CAD build for the part. Positions are in the model's coordinates, mm. A direction names the side the tool comes from. Give positions to 0.01 mm unless a question says otherwise; leave off trailing zeros. Write each loop counter-clockwise with the first axis right and the second up, starting at its lowest first coordinate (ties: lowest second). Pieces come first, ordered by that corner, then holes. Notation, with made-up numbers: (84.25, 79.5) -> (137.25, 79.5) arc R36 cw to (137.25, 115.5) -> close; hole circle Ø9 at (11, -33). An arc over 180 degrees is marked (long way). Answer as a JSON object with one key per item and string values.
```python
from build123d import *

# Parameters (mm, degrees)
F1_DEPTH = 20
F3_DEPTH = 3
F4_R     = 1


with BuildPart() as f1:
    # F0 (on Top) → F1 (new body)
    with BuildSketch(Plane.XY):
        with BuildLine():
            ThreePointArc((-22.105041, 11.299526), (-27.279634, -7.687217), (-7.672847, -6))
            Line((-7.672847, -6), (7.672847, -6))
            ThreePointArc((7.672847, -6), (27.279634, -7.687217), (22.105041, 11.299526))
            ThreePointArc((22.105041, 11.299526), (18.842402, 11.974802), (15.519847, 11.726953))
            ThreePointArc((15.519847, 11.726953), (10.990907, 9.693042), (7.672847, 6))
            Line((7.672847, 6), (-1.3, 6))
            Line((-1.3, 6), (-7.672847, 6))
            ThreePointArc((-7.672847, 6), (-10.990907, 9.693042), (-15.519847, 11.726953))
            ThreePointArc((-15.519847, 11.726953), (-18.842402, 11.974802), (-22.105041, 11.299526))
        make_face()
        with BuildLine():
            Line((-8.9, 4), (0, 4))
            Line((0, 4), (8.9, 4))
            ThreePointArc((8.9, 4), (28.065151, 0), (8.9, -4))
            Line((8.9, -4), (-8.9, -4))
            ThreePointArc((-8.9, -4), (-28.065151, 0), (-8.9, 4))
        make_face(mode=Mode.SUBTRACT)
        with BuildLine():
            ThreePointArc((22.105041, 11.299526), (0, 15.132305), (-22.105041, 11.299526))
            ThreePointArc((-22.105041, 11.299526), (-18.842402, 11.974802), (-15.519847, 11.726953))
            ThreePointArc((-15.519847, 11.726953), (0, 13.632305), (15.519847, 11.726953))
            ThreePointArc((15.519847, 11.726953), (18.842402, 11.974802), (22.105041, 11.299526))
        make_face()
    extrude(amount=F1_DEPTH)

    # F2 (on face) → F3 (join)
    with BuildSketch(Plane.XZ.offset(6)):
        Polygon((1.5, 20), (0, 20), (-1.5, 20), (-1.5, 0), (0, 0), (1.5, 0), align=None)
    extrude(amount=F3_DEPTH)

    # F4
    f4_edges = [f1.edges().sort_by_distance(p)[0] for p in [
        (1.5, -9, 10),
        (-1.5, -9, 10),
    ]]
    fillet(f4_edges, radius=F4_R)


solid = f1.part
```
1) Slice it at C-C (z = 9.25). List the corners of the cut face in (x, y), then the cut area to 3 significant figures.
Model answer:
{"outline": "(-22.11, 11.3) arc R12 ccw (long way) to (-7.67, -6) -> (-1.5, -6) -> (-1.5, -8) arc R1 ccw to (-0.5, -9) -> (0.5, -9) arc R1 ccw to (1.5, -8) -> (1.5, -6) -> (7.67, -6) arc R12 ccw (long way) to (22.11, 11.3) arc R65.66 ccw to start; hole (-15.52, 11.73) arc R12 cw to (-7.67, 6) -> (7.67, 6) arc R12 cw to (15.52, 11.73) arc R64.16 ccw to start; hole (-8.9, -4) -> (8.9, -4) arc R10 ccw (long way) to (8.9, 4) -> (-8.9, 4) arc R10 ccw (long way) to start", "area": "364 mm2"}
2) Slice it at D-D (y = -5). List the corners of the cut face in (x, z), then the cut area to 3 significant figures.
Model answer:
{"outline": "(-28.97, 0) -> (-26.73, 0) -> (-26.73, 20) -> (-28.97, 20) -> close; (-9.4, 0) -> (9.4, 0) -> (9.4, 20) -> (-9.4, 20) -> close; (26.73, 0) -> (28.97, 0) -> (28.97, 20) -> (26.73, 20) -> close", "area": "466 mm2"}
3) Slice it at B-B (x = 6). List the corners of the cut face in (y, z).
Model answer:
{"outline": "(-6, 0) -> (-4, 0) -> (-4, 20) -> (-6, 20) -> close; (4, 0) -> (6, 0) -> (6, 20) -> (4, 20) -> close; (13.35, 0) -> (14.86, 0) -> (14.86, 20) -> (13.35, 20) -> close"}
4) Mould opens along Y. For faces 4 (the cylindrical face through (-27.48, -7.44, 9.86)), 5 (the flat face through (5, -6, 10)), 6 (the flat face through (0, -4, 10)), 7 (the flat face through (0, 5, 0)) say: released by +Y, released by -Y, zero draft, split by the parting line, or undercut.
Model answer:
{"face 4": "split by the parting line", "face 5": "released by -Y", "face 6": "undercut", "face 7": "zero draft"}
5) Pin check, flat tips, straight feed: pin 1 (16 mm diameter, centred on x = -18.07, y = 0, fed in from +Z); pin 2 (6 mm diameter, centred on y = 6, z = 16.5, fed in from -X); pin 3 (3 mm diameter, centred on x = -10.5, z = 12.5, fed in from +Y); pin 4 (2 mm diameter, centred on y = -7.5, z = 8.5, fed in from -X). Stop position of each tip, or through.
Model answer:
{"pin 1": "passes through", "pin 2": "stops at x = -29.68", "pin 3": "stops at y = 14.51", "pin 4": "stops at x = -28.15"}
6) 3-axis set-ups, long thin cutter, end or side, ignore diameter. For faces 1 (the flat face through (0, 5, 20)), 2 (the flat face through (0, 4, 10)), 3 (the flat face through (-1.5, -7, 10)): which of +Z, -Z, +X, -X, +Y, -Y reach the whole face in a straight line?
Model answer:
{"face 1": "+Z, +X, -X, +Y, -Y", "face 2": "+Z, -Z", "face 3": "+Z, -Z, -Y"}
7) Slice it at A-A (y = 0). List the corners of the cut face in (x, z).
Model answer:
{"outline": "(-30.07, 0) -> (-28.07, 0) -> (-28.07, 20) -> (-30.07, 20) -> close; (28.07, 0) -> (30.07, 0) -> (30.07, 20) -> (28.07, 20) -> close"}
8) Wall check: probe 1 along X at (y, z) = (0, 14); probe 2 along Y at (x, z) = (9, 18.5); probe 3 along Y at (x, z) = (-12, 4.75). Give the ranges that are in metal, low to high.
Model answer:
{"probe 1": "x = -30.07 to -28.07, 28.07 to 30.07", "probe 2": "y = -7.86 to -4.22, 4.22 to 7.86, 13 to 14.51", "probe 3": "y = -10.35 to -7.95, 7.95 to 10.35, 12.5 to 14.03"}
